CAD build for the part. Positions are in the model's coordinates, mm. A direction names the side the tool comes from. Give positions to 0.01 mm unless a question says otherwise; leave off trailing zeros. Loops run counter-clockwise (first coordinate to the right, second up) from the corner with the lowest first, then second, coordinate; pieces in that order, holes last. Notation, with made-up numbers: M 88.25,43 L 125.25,43 A30 cw 125.25,77 Z; hole C 87,-38.75 d1. An arc over 180 degrees is marked long. Answer as CSV lines item,"result".
from build123d import *

# Parameters (mm, degrees)
BOSS_EXTRUDE4_REACH     = 119.463
BOSS_EXTRUDE4_START     = -13
SKETCH2_R               = 15
BOSS_EXTRUDE5_REACH     = 119.463
BOSS_EXTRUDE5_START     = 13
SKETCH2_3_R             = 15
CUT_EXTRUDE2_DEPTH      = 50
CUT_EXTRUDE2_DEPTH_BACK = 50
SKETCH4_R               = 11


with BuildPart() as part:
    # Sketch1 → Revolve1 (revolve)
    with BuildSketch(Plane.XY, mode=Mode.PRIVATE) as revolve1_sk:
        with BuildLine():
            Line((32.5, 0), (37.5, 0))
            Line((37.5, 0), (37.5, 72))
            Line((37.5, 72), (32.5, 72))
            Line((32.5, 72), (32.5, 75))
            Line((32.5, 75), (37.5, 75))
            Line((37.5, 75), (37.5, 78))
            Line((37.5, 78), (32.5, 78))
            Line((32.5, 78), (32.5, 81))
            Line((32.5, 81), (37.5, 81))
            Line((37.5, 81), (37.5, 84))
            Line((37.5, 84), (32.5, 84))
            Line((32.5, 84), (32.5, 87))
            Line((32.5, 87), (37.5, 87))
            Line((37.5, 87), (37.5, 90))
            Line((37.5, 90), (0, 90))
            Line((0, 90), (0, 85))
            Line((0, 85), (17.5, 85))
            ThreePointArc((17.5, 85), (24.571067812, 82.071067812), (27.5, 75))
            Line((27.5, 75), (27.5, 48))
            Line((27.5, 48), (32.5, 48))
            Line((32.5, 48), (32.5, 0))
        make_face()
    revolve(revolve1_sk.sketch.rotate(Axis((0, 0, 0), (0, 1, 0)), 90), axis=Axis((0, 0, 0), (0, 1, 0)))

    # Sketch2 → Boss-Extrude4 (add, up to next)
    with BuildSketch(Plane.XY.offset(BOSS_EXTRUDE4_START), mode=Mode.PRIVATE) as boss_extrude4_sk1:
        with Locations((0, 48)):
            Circle(SKETCH2_R)
    boss_extrude4_tool1 = extrude(boss_extrude4_sk1.sketch, amount=-BOSS_EXTRUDE4_REACH, mode=Mode.PRIVATE) - part.part
    add(boss_extrude4_tool1.solids().sort_by_distance((0, 48, -13))[0])

    # Sketch2_3 → Boss-Extrude5 (add, up to next)
    with BuildSketch(Plane.XY.offset(BOSS_EXTRUDE5_START), mode=Mode.PRIVATE) as boss_extrude5_sk1:
        with Locations((0, 48)):
            Circle(SKETCH2_3_R)
    boss_extrude5_tool1 = extrude(boss_extrude5_sk1.sketch, amount=BOSS_EXTRUDE5_REACH, mode=Mode.PRIVATE) - part.part
    add(boss_extrude5_tool1.solids().sort_by_distance((0, 48, 13))[0])

    # Sketch4 → Cut-Extrude2 (cut, two sides: drawn at the far end of the back side and taken through both)
    with BuildSketch(Plane.XY.offset(-CUT_EXTRUDE2_DEPTH_BACK)):
        with Locations(Location((0, 48, 0), (0, 0, 180))):
            Circle(SKETCH4_R)
    extrude(amount=CUT_EXTRUDE2_DEPTH + CUT_EXTRUDE2_DEPTH_BACK, mode=Mode.SUBTRACT)


solid = part.part
1) Band-saw the part on B-B on y = 22.5. Give the cut face in (x, z).
Answer below:
outline,"C 0,0 d75; hole C 0,0 d65"
2) Drill centre lines: line 1 (Y direction, x = 32.5, z = -4.5); line 2 (Y direction, x = 9, z = 33); line 3 (Y direction, x = -6, z = -23.5). Where is each one in solid material? Low to high. Write a range as from..to.
Answer below:
line 1,"y = 0..72, 75..78, 81..84, 87..90"
line 2,"y = 0..41.68, 54.32..72, 75..78, 81..84, 87..90"
line 3,"y = 34.25..38.78, 57.22..61.75, 82.37..90"
3) Band-saw the part on A-A on x = 0. Give the number of separate pieces and of enclosed holes in the cut face, and give its area (3 significant figures).
Answer below:
separate pieces,"3"
enclosed holes,"0"
area,"1,490 mm^2"
4) Mould opens along Z. For faces 4 (the face through (-1.43, 23.66, 32.47)), 5 (the face through (-28, 48, 0)), 6 (the face through (-11.26, 36.5, -35.77)), 7 (the face through (-31, 81, -11)) say: +Z half, -Z half, draft (parallel to the pull), parting line (faces both ways), or undercut.
Answer below:
face 4,"undercut"
face 5,"undercut"
face 6,"parting line"
face 7,"draft"
5) Which spindle directions (+Z, -Z, +X, -X, +Y, -Y) get a long thin tool onto all of the face, cutting with end or side? Do faces 1 (the face through (-5, 58, 13)), 2 (the face through (-31, 78, 11)), 3 (the face through (-1, 90, 1)). Say none if no direction does.
Answer below:
face 1,"-Y"
face 2,"none"
face 3,"+Z, -Z, +X, -X, +Y"
6) Flat gauge pins, fed straight in: pin 1 (1.5 mm diameter, centred on x = 9, z = 24, fed in from -Y); pin 2 (22.5 mm diameter, centred on x = 7.5, z = -16, fed in from -Y); pin 3 (8 mm diameter, centred on x = -6, y = 33, fed in from +Z). Where does each tip first touch, or does it go through?
Answer below:
pin 1,"stops at y = 35.47"
pin 2,"stops at y = 33"
pin 3,"stops at z = 37.45"
